Read the model definition and answer for the solid it produces. Units are mm, in the model's axes. Face numbers are marked on the shaded views. Coordinates: 2 decimals unless noted, no trailing zeros. Order: outer loops, then holes, each group sorted by start corner. A loop starts at its lowest first (then second) coordinate and runs counter-clockwise, first axis right, second up.
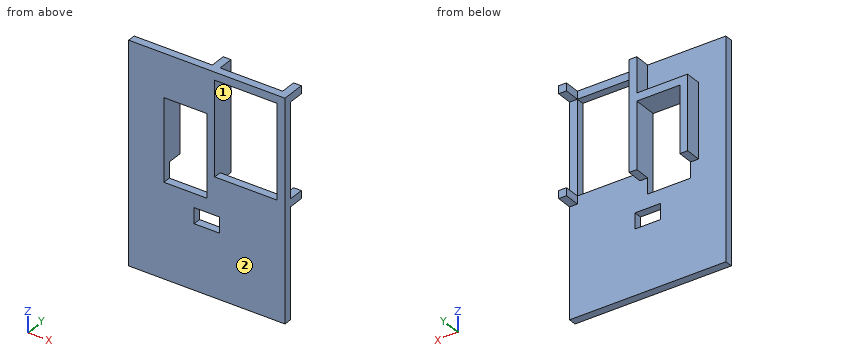
Autodesk Inventor part; units mm, degrees
ref_plane "YZ Plane" through (0, 0, 0) normal (1, 0, 0) x (0, 1, 0)
ref_plane "XZ Plane" through (0, 0, 0) normal (0, 1, 0) x (-1, 0, 0)
ref_plane "XY Plane" through (0, 0, 0) normal (0, 0, 1) x (1, 0, 0)
sketch "Sketch1" plane through (0, 0, 0) normal (0, 1, 0) x (-1, 0, 0)
  line L0 (63.5, 88.9) -> (-63.5, 88.9)
  line L1 (-63.5, 88.9) -> (-63.5, -88.9)
  line L2 (-63.5, -88.9) -> (63.5, -88.9)
  line L3 (63.5, -88.9) -> (63.5, 88.9)
  line L4 (63.5, 88.9) -> (-63.5, -88.9) construction
  line L5 (-63.5, 88.9) -> (63.5, -88.9) construction
  point P0 (0, 0)
  dimension "d0" = 177.8
  dimension "d1" = 127
extrude "main plate" add sketch "Sketch1" along normal blind 6.35
sketch "Sketch4" plane through (0, 6.35, 0) normal (0, 1, 0) x (1, 0, 0)
  line L0 (63.5, -88.9) -> (63.5, 88.9)
  line L1 (63.5, -88.9) -> (57.15, -88.9)
  line L2 (57.15, -88.9) -> (57.15, -82.55)
  line L3 (57.15, -82.55) -> (63.5, -82.55)
  line L4 (63.5, -82.55) -> (63.5, -88.9)
  line L5 (57.15, -82.55) -> (6.35, -82.55) construction
  line L6 (57.15, -82.55) -> (57.15, -6.35) construction
  line L7 (57.15, -6.35) -> (63.5, -6.35)
  line L8 (63.5, -6.35) -> (63.5, 0)
  line L9 (63.5, 0) -> (57.15, 0)
  line L10 (57.15, 0) -> (57.15, -6.35)
  line L11 (-63.5, -88.9) -> (63.5, -88.9)
  line L12 (6.35, -82.55) -> (0, -82.55)
  line L13 (0, -82.55) -> (0, -88.9)
  line L14 (0, -88.9) -> (6.35, -88.9)
  line L15 (6.35, -88.9) -> (6.35, -82.55)
  line L16 (0, 0) -> (6.35, 0)
  line L17 (6.35, 0) -> (6.35, -6.35)
  line L18 (6.35, -6.35) -> (0, -6.35)
  line L19 (0, -6.35) -> (0, 0)
  line L20 (6.35, -6.35) -> (0, -6.35)
  line L21 (0, -6.35) -> (0, -82.55)
  line L22 (0, -82.55) -> (6.35, -82.55)
  line L23 (6.35, -82.55) -> (6.35, -6.35)
  dimension "d12" = 6.35
  dimension "d13" = 6.35
  dimension "d14" = 50.8
  dimension "d15" = 76.2
extrude "battery standoffs" add sketch "Sketch4" along normal blind 12.7
sketch "Sketch5" plane through (0, 6.35, 0) normal (0, 1, 0) x (1, 0, 0)
  line L0 (-34.925, -6.35) -> (0, -6.35)
  line L1 (0, -6.35) -> (0, -53.975)
  line L2 (0, -53.975) -> (-34.925, -53.975)
  line L3 (-34.925, -53.975) -> (-34.925, -6.35)
  line L4 (-34.925, -6.35) -> (0, -6.35)
  line L5 (0, -6.35) -> (0, -53.975)
  line L6 (0, -53.975) -> (-34.925, -53.975)
  line L7 (-34.925, -53.975) -> (-34.925, -6.35)
  point P0 (0, 0)
  dimension "d18" = 34.925
  dimension "d19" = 47.625
extrude "breadboard hole" cut sketch "Sketch5" against normal blind 6.35
sketch "Sketch6" plane through (0, 6.35, 0) normal (0, 1, 0) x (1, 0, 0)
  line L0 (6.35, 0) -> (6.35, -6.35)
  line L1 (6.35, -6.35) -> (57.15, -6.35)
  line L2 (57.15, -6.35) -> (57.15, -82.55)
  line L3 (57.15, -82.55) -> (6.35, -82.55)
  line L4 (6.35, -82.55) -> (6.35, -6.35)
  point P0 (0, 0)
extrude "battery hole" cut sketch "Sketch6" against normal blind 6.35
sketch "Sketch9" plane through (0, 6.35, 0) normal (0, 1, 0) x (1, 0, 0)
  line L0 (0, -53.975) -> (0, -6.35)
  line L1 (0, -53.975) -> (-34.925, -53.975)
  line L2 (-34.925, -53.975) -> (-34.925, -60.325)
  line L3 (-34.925, -60.325) -> (0, -60.325)
  line L4 (0, -60.325) -> (0, -53.975)
  line L5 (-34.925, -60.325) -> (-41.275, -60.325)
  line L6 (-41.275, -60.325) -> (-41.275, 0)
  line L7 (-41.275, 0) -> (-34.925, 0)
  line L8 (-34.925, 0) -> (-34.925, -60.325)
  line L9 (0, 0) -> (0, -6.35)
  line L10 (-34.925, -6.35) -> (-34.925, 0)
  point P0 (0, 0)
extrude "breadboard standoffs" add sketch "Sketch9" along normal blind 12.7
sketch "Sketch10" plane through (0, 6.35, 0) normal (0, 1, 0) x (1, 0, 0)
  line L0 (-34.925, 0) -> (-34.925, -6.35)
  line L1 (-34.925, -6.35) -> (0, -6.35)
  line L2 (0, -6.35) -> (0, 12.7)
  line L3 (0, 12.7) -> (-34.925, 12.7)
  line L4 (-34.925, 12.7) -> (-34.925, -6.35)
  point P0 (0, 0)
extrude "wiring hole" cut sketch "Sketch10" against normal blind 6.35
sketch "Sketch11" plane through (0, 6.35, 0) normal (0, 1, 0) x (1, 0, 0)
  line L0 (-10.3188, 36.5125) -> (10.3187, 36.5125)
  line L1 (10.3187, 36.5125) -> (10.3187, 23.8125)
  line L2 (10.3187, 23.8125) -> (-10.3187, 23.8125)
  line L3 (-10.3187, 23.8125) -> (-10.3188, 36.5125)
  line L4 (-10.3188, 36.5125) -> (10.3187, 23.8125) construction
  line L5 (10.3187, 36.5125) -> (-10.3187, 23.8125) construction
  point P0 (0, 0)
  point P1 (0, 30.1625)
  dimension "d28" = 12.7
  dimension "d29" = 20.6375
extrude "power switch mount" cut sketch "Sketch11" against normal blind 6.35
properties part number "chassis_top"
1) A cutting plane is placed at A-A, the plane z = -5. Determine the outline of the cut face in (x, y) (3 decimals).
A:
outline: (-63.5, 0) - (-34.925, 0) - (-34.925, 6.35) - (-63.5, 6.35) - close; (0, 0) - (63.5, 0) - (63.5, 6.35) - (0, 6.35) - close
2) Straight lines are drawn through the part: line 1 (X direction, y = 7, z = 3) (3 decimals); line 2 (Z direction, x = -8, y = 3) (1 decimal); line 3 (Z direction, x = -32, y = 2.5) (3 decimals). For each, find the intervals that lie inside material, in ascending order.
A:
line 1: x = -41.275 to -34.925, 0 to 6.35, 57.15 to 63.5
line 2: z = -88.9 to -36.5, -23.8 to -12.7, 54 to 88.9
line 3: z = -88.9 to -12.7, 53.975 to 88.9
3) A cutting plane is placed at B-B, the plane x = -2. State how many separate pieces and enclosed holes the cut face has, and give its area (3 significant figures).
A:
separate pieces: 3
enclosed holes: 0
area: 706 mm2
4) A cutting plane is placed at D-D, the plane x = 16.5. Determine the outline of the cut face in (y, z).
A:
outline: (0, -88.9) - (6.35, -88.9) - (6.35, 6.35) - (0, 6.35) - close; (0, 82.55) - (6.35, 82.55) - (6.35, 88.9) - (0, 88.9) - close
5) Flat-ended cylindrical pins translate along their axes: pin 1 Ø3 at (x, z) = (5, -63.5) entering from +Y; pin 2 Ø3 at (x, y) = (-28, 15.5) entering from +Z (3 decimals); pin 3 Ø5 at (x, y) = (60.5, 13.5) entering from -Z. Find the tip coordinate at first contact, or state that the pin passes through.
A:
pin 1: stops at y = 6.35
pin 2: stops at z = 60.325
pin 3: stops at z = 0
6) Determine the mould class of the marked faces 1 and 2 for opening direction Z: pulls with the +Z half, pulls with the -Z half, needs draft (parallel to the pull), parting line crosses it, or undercut.
A:
face 1: undercut
face 2: needs draft
